Autodesk Inventor part; units mm, degrees
ref_plane "YZ Plane" through (0, 0, 0) normal (1, 0, 0) x (0, 1, 0)
ref_plane "XZ Plane" through (0, 0, 0) normal (0, 1, 0) x (-1, 0, 0)
ref_plane "XY Plane" through (0, 0, 0) normal (0, 0, 1) x (1, 0, 0)
sketch "Sketch1" plane through (0, 0, 0) normal (0, 0, 1) x (1, 0, 0)
  line L0 (0, 0) -> (20, 0)
  line L1 (20, 0) -> (20, 22.2)
  line L2 (20, 22.2) -> (0, 22.2)
  line L3 (0, 22.2) -> (0, 0)
  dimension "d0" = 20
  dimension "d1" = 22.2
extrude "Extrusion1" add sketch "Sketch1" along normal mid plane 12.2
sketch "Sketch2" plane through (0, 0, 6.1) normal (-1, 0, 0) x (0, 0, 1)
  circle A0 centre (-6, 6) radius 6
  line L0 (0, 0) -> (-12.2, 0)
  line L1 (0, 22.2) -> (0, 0)
  point P0 (-6.1, 0)
  dimension "d4" = 6
  dimension "d5" = 6
  dimension "d6" = 12
extrude "Extrusion2" add sketch "Sketch2" along normal blind 3 contours A0
sketch "Sketch3" plane through (0, 22.2, 6.1) normal (0, 1, 0) x (1, 0, 0)
  line L0 (0, 0) -> (20, 0)
  line L1 (3, 12.2) -> (4.3, 12.2)
  line L2 (4.3, 12.2) -> (4.3, 0)
  line L3 (4.3, 0) -> (3, 0)
  line L4 (3, 0) -> (3, 12.2)
  line L5 (0, 12.2) -> (0, 0)
  point P0 (0, 6.1)
  dimension "d9" = 3
  dimension "d10" = 1.3
  dimension "d11" = 12.2
extrude "Extrusion3" add sketch "Sketch3" along normal blind 5 and the other way blind 27.2
sketch "Sketch5" plane through (4.3, -5, 6.1) normal (1, 0, 0) x (0, 0, -1)
  line L0 (0, 0) -> (12.2, 0)
  line L1 (12.2, 0) -> (12.2, 4)
  line L2 (12.2, 4) -> (0, 4)
  line L3 (0, 4) -> (0, 0)
  line L4 (0, 5) -> (0, 0)
  line L5 (12.2, 5) -> (12.2, 0)
  line L6 (12.2, 0) -> (0, 0)
  line L7 (12.2, 5) -> (0, 5)
  point P0 (6.1, 5)
  dimension "d24" = 1
extrude "Extrusion5" cut sketch "Sketch5" against normal blind 2 contours L3 L2 L1 L0
properties part number "Servo"
Input: part model. Units: mm. Frame: model coordinates. A direction names the side the tool comes from. Round coordinates to 2 decimals unless told otherwise and drop trailing zeros. Loops run counter-clockwise (first coordinate to the right, second up) from the corner with the lowest first, then second, coordinate; pieces in that order, holes last. Notation, with made-up numbers: (6, 0.25) - (47, 0.25) arc R27 ccw to (47, 22.25) - close; hole circle Ø1 at (7, 39.25). An arc over 180 degrees is marked (long way). One line per item, written item: value. Start each with the question number.
(1) Section B-B, the plane y = 9.5. Return loops of the section in (x, z), plus the area to 3 significant figures.
(2) Ray query, line 1 (X direction, y = 16.25, z = 1.5); line 2 (Y direction, x = 5.25, z = 1.75); line 3 (X direction, y = 25.25, z = 0.75). Return the intervals inside material, ascending. Write a range as [from, to].
(3) Section C-C, the plane x = 16.5. Return loops of the section in (y, z).
(4) Contact query for flat-ended pins moving along their axis: P1, Ø1.5, axis at x = 1.5, z = -1.5, coming from the -Y side; P2, Ø0.9, axis at x = 1.5, z = -2, coming from the +Y side; P3, Ø0.8, axis at y = -0.5, z = -2.5, coming from the -X side. Output: stop coordinate, or through.
(5) Section A-A, the plane z = -3.5. Return loops of the section in (x, y), plus the area to 3 significant figures.
(6) Access query for faces 1 (the flat face through (3, -0.5, 0.1)), 2 (the flat face through (4.3, -0.5, -0.1)), 3 (the cylindrical face through (-1.48, 8.3, 5.64)). Directions: +Z, -Z, +X, -X, +Y, -Y. A direction counts if a zero-diameter tool reaches every point of the face in a straight line with its end or side. Return the directions, or none.
Results below:
1. outline: (-3, -4.77) - (0, -4.77) - (0, -6.1) - (20, -6.1) - (20, 6.1) - (0, 6.1) - (0, 4.97) - (-3, 4.97) - close
1. area: 273 mm^2
2. line 1: [0, 20]
2. line 2: [0, 22.2]
2. line 3: [3, 4.3]
3. outline: (0, -6.1) - (22.2, -6.1) - (22.2, 6.1) - (0, 6.1) - close
4. P1: y = 0
4. P2: y = 22.2
4. P3: x = 3
5. outline: (-3, 1.2) - (0, 1.2) - (0, 0) - (3, 0) - (3, -1) - (4.3, -1) - (4.3, 0) - (20, 0) - (20, 22.2) - (4.3, 22.2) - (4.3, 27.2) - (3, 27.2) - (3, 22.2) - (0, 22.2) - (0, 10.8) - (-3, 10.8) - close
5. area: 481 mm^2
6. face 1: +Z, -Z, -X, -Y
6. face 2: +Z, -Z, +X, -Y
6. face 3: -X
